Model file for the job. Use its own axes, mm. A direction names the side the tool comes from. Give positions to 0.01 mm unless a question says otherwise; leave off trailing zeros. Loops run counter-clockwise (first coordinate to the right, second up) from the corner with the lowest first, then second, coordinate; pieces in that order, holes last. Notation, with made-up numbers: (2.25, 68) -> (50.25, 68) arc R26 ccw to (50.25, 107) -> close; hole circle Ø5 at (75, -31.5). An arc over 180 degrees is marked (long way). Use CSV: the item, a comma, the result in double quotes. Start each with the question number.
(1) Drill centre lines: probe 1 along X at (y, z) = (-2.75, 46); probe 2 along X at (y, z) = (-4.25, 46); probe 3 along Y at (x, z) = (0, 56.2). Where is each one in solid material? Low to high.
(2) Flat gauge pins, fed straight in: pin 1 (3 mm diameter, centred on y = 21.5, z = 52, fed in from -X); pin 2 (4 mm diameter, centred on y = 19, z = 53.5, fed in from +X); pin 3 (0.9 mm diameter, centred on y = 10, z = 57, fed in from -X); pin 4 (4 mm diameter, centred on x = -11.5, y = 2.5, fed in from -Z). Where does each tip first touch, or does it go through?
(3) 3-axis set-ups, long thin cutter, end or side, ignore diameter. For faces 1 (the flat face through (14.5, 14, 57)), 2 (the cylindrical face through (-21.51, -4.77, 43.5)), 3 (the flat face through (-6.5, 2, 56)), 4 (the flat face through (-7, 24, 55)): which of +Z, -Z, +X, -X, +Y, -Y reach the whole face in a straight line?
(4) Cut at A-A on x = 0. Write the cut outline in (y, z).
(5) Cut at B-B on y = 14.5. Write the cut outline in (x, z).
(6) Cut at D-D on y = 2.5. Write the cut outline in (x, z), then the cut area to 3 significant figures.
(7) Pull direction Z, two halves, no side cores. Call faces 5 (the cylindrical face through (19.734, -4.775, 42.853)), 6 (the cylindrical face through (-20.63, -3.25, 44.65)), 7 (the flat face through (14.596, -1, 49)), 8 (the cylindrical face through (0, -1, 55)): pulls with the +Z half, pulls with the -Z half, needs draft (parallel to the pull), parting line crosses it, or undercut.
(8) Cut at C-C on z = 45. Write the cut outline in (x, y), then the cut area to 3 significant figures.
from build123d import *

# Parameters (mm, degrees)
SKETCH1_R           = 1.7
BOSS_EXTRUDE2_DEPTH = 3
SKETCH1_7_W         = 29
SKETCH1_7_H         = 3
BOSS_EXTRUDE4_DEPTH = 29
CUT_EXTRUDE1_REACH  = 43.653
SKETCH2_R           = 1.2
BOSS_EXTRUDE3_START = -3
SKETCH1_5_R         = 3.15
SKETCH1_5_R_2       = 1.7
BOSS_EXTRUDE3_DEPTH = 3.6


with BuildPart() as part:
    # Sketch1 → Boss-Extrude2 (new body)
    with BuildSketch(Plane(origin=(0, 0, 0), x_dir=(1, 0, 0), z_dir=(0, 1, 0))):
        with BuildLine():
            ThreePointArc((24.595917942, -46), (19.595917942, -41), (14.595917942, -46))
            Line((14.595917942, -46), (14.595917942, -53.027909439))
            ThreePointArc((14.595917942, -53.027909439), (0, -55), (-14.595917942, -53.027909439))
            Line((-14.595917942, -53.027909439), (-14.595917942, -46))
            ThreePointArc((-14.595917942, -46), (-19.595917942, -41), (-24.595917942, -46))
            Line((-24.595917942, -46), (-24.595917942, -58))
            Line((-24.595917942, -58), (24.595917942, -58))
            Line((24.595917942, -58), (24.595917942, -46))
        make_face()
        with Locations(Location((-19.595917942, -46, 0), (0, 0, 270))):
            Circle(SKETCH1_R, mode=Mode.SUBTRACT)
        with Locations(Location((19.595917942, -46, 0), (0, 0, 270))):
            Circle(SKETCH1_R, mode=Mode.SUBTRACT)
    extrude(amount=-BOSS_EXTRUDE2_DEPTH)

    # Sketch1<7> → Boss-Extrude4 (add)
    with BuildSketch(Plane(origin=(0, 0, 0), x_dir=(1, 0, 0), z_dir=(0, 1, 0))):
        with Locations((0, -56.5)):
            Rectangle(SKETCH1_7_W, SKETCH1_7_H)
    extrude(amount=BOSS_EXTRUDE4_DEPTH)

    # Sketch2 → Cut-Extrude1 (cut, up to next)
    with BuildSketch(Plane.XY.offset(58), mode=Mode.PRIVATE) as cut_extrude1_sk1:
        with BuildLine():
            Line((-6.5, 5.013167019), (-6.5, -0.6))
            Line((-6.5, -0.6), (6.5, -0.6))
            Line((6.5, -0.6), (6.5, 5.013167019))
            ThreePointArc((6.5, 5.013167019), (0, 26), (-6.5, 5.013167019))
        make_face()
    cut_extrude1_tool1 = extrude(cut_extrude1_sk1.sketch, amount=-CUT_EXTRUDE1_REACH, mode=Mode.PRIVATE) & part.part
    # Sketch2 → Cut-Extrude1 (cut, up to next)
    with BuildSketch(Plane.XY.offset(58), mode=Mode.PRIVATE) as cut_extrude1_sk2:
        with Locations((-11.5, 2.5)):
            Circle(SKETCH2_R)
    cut_extrude1_tool2 = extrude(cut_extrude1_sk2.sketch, amount=-CUT_EXTRUDE1_REACH, mode=Mode.PRIVATE) & part.part
    # Sketch2 → Cut-Extrude1 (cut, up to next)
    with BuildSketch(Plane.XY.offset(58), mode=Mode.PRIVATE) as cut_extrude1_sk3:
        with Locations((-11.5, 26.5)):
            Circle(SKETCH2_R)
    cut_extrude1_tool3 = extrude(cut_extrude1_sk3.sketch, amount=-CUT_EXTRUDE1_REACH, mode=Mode.PRIVATE) & part.part
    # Sketch2 → Cut-Extrude1 (cut, up to next)
    with BuildSketch(Plane.XY.offset(58), mode=Mode.PRIVATE) as cut_extrude1_sk4:
        with Locations((11.5, 2.5)):
            Circle(SKETCH2_R)
    cut_extrude1_tool4 = extrude(cut_extrude1_sk4.sketch, amount=-CUT_EXTRUDE1_REACH, mode=Mode.PRIVATE) & part.part
    # Sketch2 → Cut-Extrude1 (cut, up to next)
    with BuildSketch(Plane.XY.offset(58), mode=Mode.PRIVATE) as cut_extrude1_sk5:
        with Locations((11.5, 26.5)):
            Circle(SKETCH2_R)
    cut_extrude1_tool5 = extrude(cut_extrude1_sk5.sketch, amount=-CUT_EXTRUDE1_REACH, mode=Mode.PRIVATE) & part.part
    add(cut_extrude1_tool1.solids().sort_by_distance((0, 12.98305, 58))[0], mode=Mode.SUBTRACT)
    add(cut_extrude1_tool2.solids().sort_by_distance((-11.5, 2.5, 58))[0], mode=Mode.SUBTRACT)
    add(cut_extrude1_tool3.solids().sort_by_distance((-11.5, 26.5, 58))[0], mode=Mode.SUBTRACT)
    add(cut_extrude1_tool4.solids().sort_by_distance((11.5, 2.5, 58))[0], mode=Mode.SUBTRACT)
    add(cut_extrude1_tool5.solids().sort_by_distance((11.5, 26.5, 58))[0], mode=Mode.SUBTRACT)

    # Sketch1<5> → Boss-Extrude3 (add)
    with BuildSketch(Plane(origin=(0, 0, 0), x_dir=(1, 0, 0), z_dir=(0, 1, 0)).offset(BOSS_EXTRUDE3_START)):
        with Locations(Location((-19.595917942, -46, 0), (0, 0, 270))):
            Circle(SKETCH1_5_R)
        with Locations(Location((-19.595917942, -46, 0), (0, 0, 270))):
            Circle(SKETCH1_5_R_2, mode=Mode.SUBTRACT)
        with Locations(Location((19.595917942, -46, 0), (0, 0, 270))):
            Circle(SKETCH1_5_R)
        with Locations(Location((19.595917942, -46, 0), (0, 0, 270))):
            Circle(SKETCH1_5_R_2, mode=Mode.SUBTRACT)
    extrude(amount=-BOSS_EXTRUDE3_DEPTH)


solid = part.part
Check result:
1,probe 1,"-24.6 to -21.3, -17.9 to -14.6, 14.6 to 17.9, 21.3 to 24.6"
1,probe 2,"-22.75 to -21.3, -17.9 to -16.45, 16.45 to 17.9, 21.3 to 22.75"
1,probe 3,"-3 to -0.6, 26 to 29"
2,pin 1,"through"
2,pin 2,"x = 14.5"
2,pin 3,"x = -14.5"
2,pin 4,"z = 55"
3,face 1,"+Z, -Z, +X, +Y"
3,face 2,"-Y"
3,face 3,"+Z, -Z"
3,face 4,"-Z, +X, -X, +Y"
4,outline,"(-3, 55) -> (-0.6, 55) -> (-0.6, 58) -> (-3, 58) -> close; (26, 55) -> (29, 55) -> (29, 58) -> (26, 58) -> close"
5,outline,"(-14.5, 55) -> (-11.5, 55) -> (-11.5, 58) -> (-14.5, 58) -> close; (11.5, 55) -> (14.5, 55) -> (14.5, 58) -> (11.5, 58) -> close"
6,outline,"(-14.5, 55) -> (-12.7, 55) -> (-12.7, 58) -> (-14.5, 58) -> close; (-10.3, 55) -> (-6.5, 55) -> (-6.5, 58) -> (-10.3, 58) -> close; (6.5, 55) -> (10.3, 55) -> (10.3, 58) -> (6.5, 58) -> close; (12.7, 55) -> (14.5, 55) -> (14.5, 58) -> (12.7, 58) -> close"
6,area,"33.6 mm²"
7,face 5,"parting line crosses it"
7,face 6,"undercut"
7,face 7,"needs draft"
7,face 8,"pulls with the -Z half"
8,outline,"(-24.49, -3) -> (-22.58, -3) -> (-22.58, -6.6) -> (-20.97, -6.6) -> (-20.97, 0) -> (-24.49, 0) -> close; (-18.22, -6.6) -> (-16.61, -6.6) -> (-16.61, -3) -> (-14.7, -3) -> (-14.7, 0) -> (-18.22, 0) -> close; (14.7, -3) -> (16.61, -3) -> (16.61, -6.6) -> (18.22, -6.6) -> (18.22, 0) -> (14.7, 0) -> close; (20.97, -6.6) -> (22.58, -6.6) -> (22.58, -3) -> (24.49, -3) -> (24.49, 0) -> (20.97, 0) -> close"
8,area,"65.5 mm²"
